Part model, mm, in its own coordinate system. Face numbers are marked on the shaded views. Round coordinates to 2 decimals unless told otherwise and drop trailing zeros. Write each loop counter-clockwise with the first axis right and the second up, starting at its lowest first coordinate (ties: lowest second). Pieces come first, ordered by that corner, then holes. Notation, with made-up numbers: M 81.5,63.5 L 89.5,63.5 A17 ccw 89.5,69.5 Z; hole C 36.5,17.25 d10. An arc over 180 degrees is marked long. Use one line per item in the form item = value. Start each with the question number.
Item 1: Flat gauge pins, fed straight in: pin 1 Ø6 at (y, z) = (42, 8.5) entering from +X; pin 2 Ø2 at (x, z) = (-19, 6.5) entering from +Y; pin 3 Ø2 at (x, y) = (-29.5, 51.5) entering from +Z. Where does each tip first touch, or does it go through?
Item 2: Mould opens along Y. For the marked faces 1 and 2 say: +Y half, -Y half, draft (parallel to the pull), parting line (faces both ways), or undercut.
Item 3: Cut at A-A, the plane x = -20. Give the cut face in (y, z), then the cut area to 3 significant figures.
Item 4: Cut at C-C, the plane z = 9.75. State how many separate pieces and enclosed holes the cut face has, then the cut area to 3 significant figures.
Item 5: Cut at B-B, the plane y = 36. Give the cut face in (x, z), then the cut area to 3 significant figures.
Item 6: Probe L1, parallel to Y at x = -4, z = 7.75; L2, parallel to X at y = 3, z = 11; L3, parallel to Z at x = -39.5, y = 39.5. List the from-to ranges inside material, lowest first.
Item 7: Cut at D-D, the plane x = -4. Give the cut face in (y, z).
from build123d import *

# Parameters (mm, degrees)
SKETCH1_W           = 80
SKETCH1_H           = 56
BOSS_EXTRUDE1_DEPTH = 4
SKETCH2_R           = 2.4
BOSS_EXTRUDE2_DEPTH = 8


with BuildPart() as part:
    # Sketch1 → Boss-Extrude1 (new body)
    with BuildSketch(Plane(origin=(0, 0, 0), x_dir=(0, 1, 0), z_dir=(0, 0, 1))):
        with Locations((40, 28)):
            Rectangle(SKETCH1_W, SKETCH1_H)
    extrude(amount=BOSS_EXTRUDE1_DEPTH)

    # Sketch2 → Boss-Extrude2 (add)
    with BuildSketch(Plane.XY.offset(4)):
        with Locations((-4, 4.172184478)):
            Circle(SKETCH2_R)
        with Locations((-20, 4.172184478)):
            Circle(SKETCH2_R)
        with Locations((-36, 4.172184478)):
            Circle(SKETCH2_R)
        with Locations((-52, 4.172184478)):
            Circle(SKETCH2_R)
        with Locations(Location((-52, 75.827815522, 0), (0, 0, 180))):
            Circle(SKETCH2_R)
        with Locations(Location((-36, 75.827815522, 0), (0, 0, 180))):
            Circle(SKETCH2_R)
        with Locations(Location((-20, 75.827815522, 0), (0, 0, 180))):
            Circle(SKETCH2_R)
        with Locations(Location((-4, 75.827815522, 0), (0, 0, 180))):
            Circle(SKETCH2_R)
        with Locations((-4, 36)):
            Circle(SKETCH2_R)
        with Locations(Location((-4, 44, 0), (0, 0, 180))):
            Circle(SKETCH2_R)
        with Locations((-52, 44)):
            Circle(SKETCH2_R)
        with Locations(Location((-52, 36, 0), (0, 0, 180))):
            Circle(SKETCH2_R)
    extrude(amount=BOSS_EXTRUDE2_DEPTH)


solid = part.part
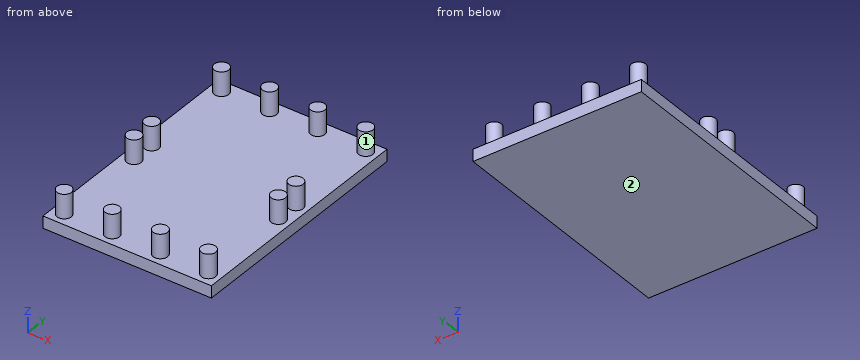
Model answer:
q1.pin_1 = -1.6
q1.pin_2 = 78.23
q1.pin_3 = 4
q2.face_1 = undercut
q2.face_2 = draft
q3.outline = M 0,0 L 80,0 L 80,4 L 78.23,4 L 78.23,12 L 73.43,12 L 73.43,4 L 6.57,4 L 6.57,12 L 1.77,12 L 1.77,4 L 0,4 Z
q3.area = 397 mm²
q4.separate_pieces = 12
q4.enclosed_holes = 0
q4.area = 217 mm²
q5.outline = M -56,0 L 0,0 L 0,4 L -1.6,4 L -1.6,12 L -6.4,12 L -6.4,4 L -49.6,4 L -49.6,12 L -54.4,12 L -54.4,4 L -56,4 Z
q5.area = 301 mm²
q6.L1 = 1.77 to 6.57, 33.6 to 38.4, 41.6 to 46.4, 73.43 to 78.23
q6.L2 = -54.09 to -49.91, -38.09 to -33.91, -22.09 to -17.91, -6.09 to -1.91
q6.L3 = 0 to 4
q7.outline = M 0,0 L 80,0 L 80,4 L 78.23,4 L 78.23,12 L 73.43,12 L 73.43,4 L 46.4,4 L 46.4,12 L 41.6,12 L 41.6,4 L 38.4,4 L 38.4,12 L 33.6,12 L 33.6,4 L 6.57,4 L 6.57,12 L 1.77,12 L 1.77,4 L 0,4 Z
